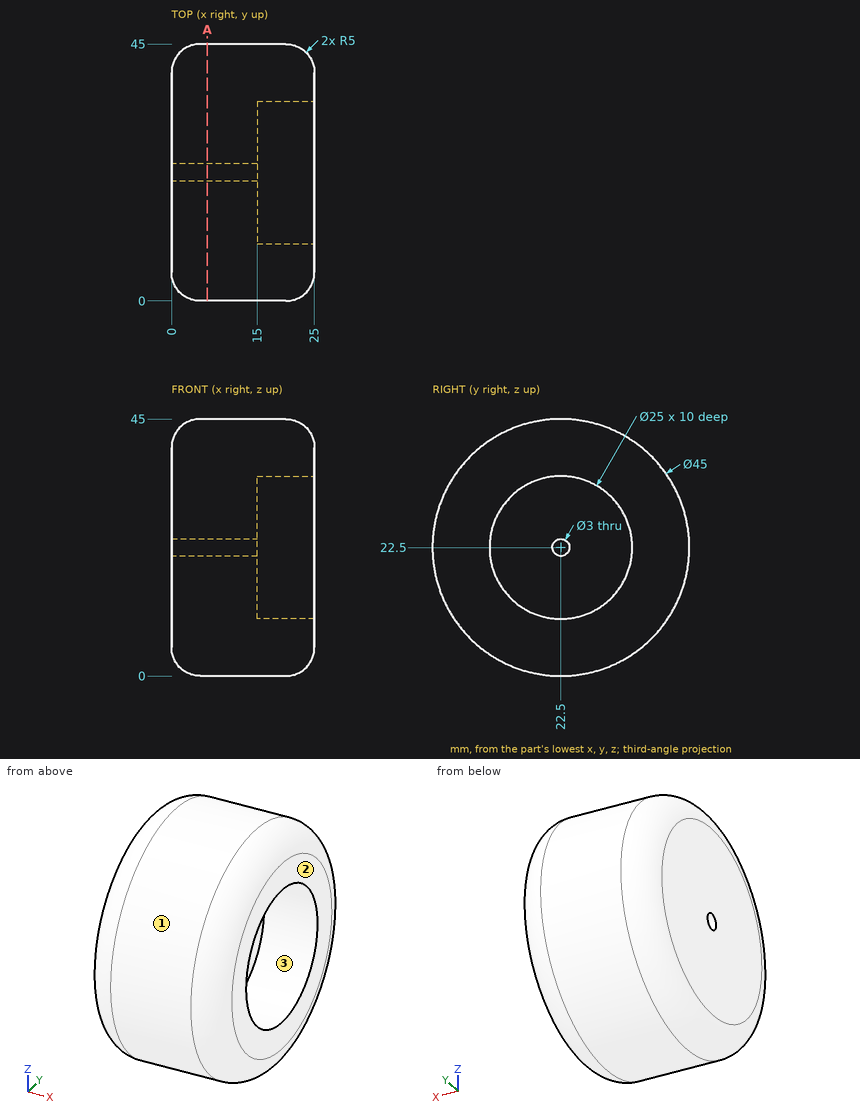
Drawing for the job (mm, zero at the part's lowest x, y, z). Round coordinates to 2 decimals unless told otherwise and drop trailing zeros. Loops run counter-clockwise (first coordinate to the right, second up) from the corner with the lowest first, then second, coordinate; pieces in that order, holes last. Notation, with made-up numbers: (76, 0.5) - (81, 0.5) arc R15 cw to (81, 17.5) - close; hole circle Ø7 at (10.25, 20.5). An arc over 180 degrees is marked (long way). Write each question's results on one line, items separated by ' | '.
(1) Pin check, flat tips, straight feed: pin 1 (3 mm diameter, centred on x = 17, y = 17, fed in from +Z); pin 2 (5 mm diameter, centred on x = 15, y = 35, fed in from +Z); pin 3 (3 mm diameter, centred on x = 15, y = 12.5, fed in from -Z). Stop position of each tip, or through.
Answer below:
pin 1: stops at z = 44.64 | pin 2: stops at z = 42.66 | pin 3: stops at z = 1.67
(2) Mould opens along Z. For the marked faces 1, 2 and 3 say: released by +Z, released by -Z, zero draft, split by the parting line, or undercut.
Answer below:
face 1: split by the parting line | face 2: zero draft | face 3: undercut
(3) Wall check: L1, parallel to Y at x = 7.75, z = 22.5; L2, parallel to X at y = 23, z = 11; L3, parallel to Y at x = 20, z = 22.5. Give the ranges that are in metal, low to high.
Answer below:
L1: y = 0 to 21, 24 to 45 | L2: x = 0 to 15 | L3: y = 0 to 10, 35 to 45
(4) Saw through at A-A, the plane x = 6.25. List the corners of the cut face in (y, z), then the cut area to 3 significant figures.
Answer below:
outline: circle Ø45 at (22.5, 22.5); hole circle Ø3 at (22.5, 22.5) | area: 1,580 mm^2
